```python
from build123d import *

# Parameters (mm, degrees)
F0_W      = 184.15
F0_H      = 50.8
F1_DEPTH  = 3.175
F3_D      = 3.2
F4_W      = 184.15
F4_H      = 3.175
F5_DEPTH  = 76.2
F7_D      = 3.3
F8_W      = 3.175
F8_H      = 47.625
F9_DEPTH  = 76.2
F10_W     = 19.05
F10_H     = 34.925
F11_DEPTH = 3.175
F12_W     = 3.175
F12_H     = 47.625
F13_DEPTH = 76.2
F14_W     = 13.2291666667
F14_H     = 31.75
F14_W_2   = 11.6416666667
F15_DEPTH = 3.175
F16_W     = 6.35
F16_H     = 6.35
F17_DEPTH = 6.35
F19_D     = 2.4
F19_DEPTH = 12.7
F19_TIP   = 0.7210327428
F20_W     = 121.4
F20_H     = 34.925
F21_DEPTH = 25.4
F22_W     = 60.2
F22_H     = 32.26
F23_DEPTH = 25.4
F24_W     = 177.8
F24_H     = 76.2
F25_DEPTH = 50.801
F26_W     = 6.35
F26_H     = 6.35
F27_DEPTH = 9.525
F28_D     = 2.4
F28_DEPTH = 12.7
F28_TIP   = 0.7210327428
F29_W     = 165.1
F29_H     = 6.35
F29_R     = 1.2
F30_DEPTH = 3.175


with BuildPart() as f1:
    # F0 (on Top) → F1 (new body)
    with BuildSketch(Plane.XY):
        with Locations((-3.8965528874, 0)):
            Rectangle(F0_W, F0_H)
    extrude(amount=F1_DEPTH)

    # F3 (through all)
    with Locations(Plane.XY.offset(3.175)):
        with Locations((-78.8965528874, 9.525), (-78.8965528874, -15.475), (71.1034471126, -15.475), (71.1034471126, 9.525)):
            Hole(F3_D / 2)

    # F4 (on face) → F5 (join)
    with BuildSketch(Plane.XY.offset(3.175)):
        with Locations((-3.8965528874, 23.8125)):
            Rectangle(F4_W, F4_H)
    extrude(amount=F5_DEPTH)

    # F7 (through all)
    with Locations(Plane.XZ.offset(-22.225)):
        with Locations((-70.5715528874, 66.675), (11.9784471126, 66.675), (10.7084471126, 18.415), (-64.2215528874, 18.415)):
            Hole(F7_D / 2)

    # F8 (on face) → F9 (join)
    with BuildSketch(Plane.XY.offset(3.175)):
        with Locations((-94.3840528874, -1.5875)):
            Rectangle(F8_W, F8_H)
    extrude(amount=F9_DEPTH)

    # F10 (on face) → F11 (cut, through all)
    with BuildSketch(Plane(origin=(-95.9715528874, 0, 0), x_dir=(0, -1, 0), z_dir=(-1, 0, 0))):
        with Locations((12.7, 58.7375)):
            Rectangle(F10_W, F10_H)
        with Locations((12.7, 20.6375)):
            Rectangle(F10_W, F10_H)
    extrude(amount=-F11_DEPTH, mode=Mode.SUBTRACT)

    # F12 (on face) → F13 (join)
    with BuildSketch(Plane.XY.offset(3.175)):
        with Locations((86.5909471126, -1.5875)):
            Rectangle(F12_W, F12_H)
    extrude(amount=F13_DEPTH)

    # F14 (on face) → F15 (cut, through all)
    with BuildSketch(Plane.YZ.offset(88.1784471126)):
        with Locations((-15.6104166667, 19.05)):
            Rectangle(F14_W, F14_H)
        with Locations((0, 19.05)):
            Rectangle(F14_W_2, F14_H)
        with Locations((15.6104166667, 19.05)):
            Rectangle(F14_W, F14_H)
    extrude(amount=-F15_DEPTH, mode=Mode.SUBTRACT)

    # F16 (on face) → F17 (join)
    with BuildSketch(Plane.XZ.offset(-22.225)):
        with Locations((-89.6215528874, 76.2)):
            Rectangle(F16_W, F16_H)
        with Locations((81.8284471126, 76.2)):
            Rectangle(F16_W, F16_H)
    extrude(amount=F17_DEPTH)

    # F19
    with Locations(Plane.XY.offset(79.375)):
        with Locations((-89.6215528874, 19.05), (81.8284471126, 19.05)):
            Hole(F19_D / 2, depth=F19_DEPTH)
            with Locations((0, 0, -(F19_DEPTH + F19_TIP / 2))):  # 118° drill point
                Cone(0, F19_D / 2, F19_TIP, mode=Mode.SUBTRACT)

    # F20 (on face) → F21 (cut)
    with BuildSketch(Plane.XY.offset(3.175)):
        with Locations((-3.8965528874, -1.5875)):
            Rectangle(F20_W, F20_H)
    extrude(amount=-F21_DEPTH, mode=Mode.SUBTRACT)

    # F22 (on face) → F23 (cut)
    with BuildSketch(Plane.XZ.offset(-22.225)):
        with Locations((-26.1215528874, 42.545)):
            Rectangle(F22_W, F22_H)
    extrude(amount=-F23_DEPTH, mode=Mode.SUBTRACT)

    # F24 (on face) → F25 (cut, through all)
    with BuildSketch(Plane.XZ.offset(25.4)):
        with Locations((-3.8965528874, 41.275)):
            Rectangle(F24_W, F24_H)
        Polygon((88.1784471126, 79.375), (85.0034471126, 79.375), (85.0034471126, 3.175), (85.0034471126, 0), (88.1784471126, 0), align=None)
    extrude(amount=-F25_DEPTH, mode=Mode.SUBTRACT)

    # F26 (on face) → F27 (join)
    with BuildSketch(Plane(origin=(0, 25.4, 0), x_dir=(-1, 0, 0), z_dir=(0, 1, 0))):
        with Locations((-81.8284471126, 6.35)):
            Rectangle(F26_W, F26_H)
        Polygon((-78.6534471126, 3.175), (-85.0034471126, 3.175), (-85.0034471126, 0), (95.9715528874, 0), (95.9715528874, 79.375), (92.7965528874, 79.375), (92.7965528874, 9.525), (92.7965528874, 3.175), (86.4465528874, 3.175), align=None)
        with Locations((89.6215528874, 6.35)):
            Rectangle(F26_W, F26_H)
    extrude(amount=-F27_DEPTH)

    # F28
    with Locations(Plane(origin=(0, 25.4, 0), x_dir=(-1, 0, 0), z_dir=(0, 1, 0))):
        with Locations((89.6215528874, 6.35), (-81.8284471126, 6.35)):
            Hole(F28_D / 2, depth=F28_DEPTH)
            with Locations((0, 0, -(F28_DEPTH + F28_TIP / 2))):  # 118° drill point
                Cone(0, F28_D / 2, F28_TIP, mode=Mode.SUBTRACT)

    # F29 (on face) → F30 (cut)
    with BuildSketch(Plane(origin=(0, 25.4, 0), x_dir=(-1, 0, 0), z_dir=(0, 1, 0))):
        with Locations((3.8965528874, 6.35)):
            Rectangle(F29_W, F29_H)
        Polygon((-78.6534471126, 9.525), (-85.0034471126, 9.525), (-85.0034471126, 2.9308686499), (92.7965528874, 2.9308686499), (92.7965528874, 9.525), (86.4465528874, 9.525), (86.4465528874, 3.175), (-78.6534471126, 3.175), align=None)
        with Locations((-81.8284471126, 6.35)):
            Circle(F29_R, mode=Mode.SUBTRACT)
        with Locations((89.6215528874, 6.35)):
            Circle(F29_R, mode=Mode.SUBTRACT)
    extrude(amount=-F30_DEPTH, mode=Mode.SUBTRACT)


solid = f1.part
```
Design review of the part built by this model. Coordinates are the model's own, in mm. A direction names the side the tool comes from. Round coordinates to 2 decimals unless told otherwise and drop trailing zeros. Write each loop counter-clockwise with the first axis right and the second up, starting at its lowest first coordinate (ties: lowest second). Pieces come first, ordered by that corner, then holes. Notation, with made-up numbers: (74, 89) -> (133, 89) arc R20 ccw to (133, 94) -> close; hole circle Ø3 at (30.5, 32). An arc over 180 degrees is marked (long way). Write item = value, one per line. Start each with the question number.
1) Clearance check with flat-ended pins moving along their axes: pin 1 (7 mm diameter, centred on x = 83, z = 7.5, fed in from -Y) (3 decimals); pin 2 (7 mm diameter, centred on x = 81, y = 18, fed in from +Z) (3 decimals); pin 3 (5 mm diameter, centred on x = -6, y = -20, fed in from +Z) (3 decimals). State where each tip first meets the part, or that it passes through.
2) Take a section at A-A, the plane y = 1. State the section outline as (x, z) points (3 decimals), plus the area to 3 significant figures.
3) Take a section at B-B, the plane z = 66. State the section outline as (x, y) points (3 decimals), plus the area to 3 significant figures.
4) Take a section at C-C, the plane y = -7.5. State the section outline as (x, z) points (3 decimals), plus the area to 3 significant figures.
5) Take a section at D-D, the plane x = -7. State the section outline as (y, z) points (3 decimals).
6) Mouldability with a two-part tool opening along Y and no side actions: class faces 1 (the face through (-94, -13, 76.2)), 2 (the face through (-5, 25.4, 2)), 3 (the face through (-46, -25.4, 1)), 4 (the face through (-90, 19, 9.525)) as +Y half, -Y half, draft (parallel to the pull), parting line (faces both ways), or undercut.
7) Tool access review of faces 5 (the face through (-90, 15.875, 5)), 6 (the face through (78.653, 19, 6)), 7 (the face through (85.003, 6, 3)), 8 (the face through (-5, 15.875, 2)), 9 (the face through (-94, -13, 41.275)): name each direction out of +Z, -Z, +X, -X, +Y, -Y from which nothing blocks a thin tool from reaching the whole face with its end or side.
8) Wall thickness on probe 1 along X at (y, z) = (17, 33.5); probe 2 along X at (y, z) = (17, 6); probe 3 along Z at (x, y) = (-68, 13) (3 decimals): over which ranges is each line inside the solid? List them lowest first. Write a range as from..to.
Results list:
q1.pin_1 = 15.875
q1.pin_2 = 9.525
q1.pin_3 = 3.175
q2.outline = (-95.972, 0) -> (-64.597, 0) -> (-64.597, 3.175) -> (-92.797, 3.175) -> (-92.797, 79.375) -> (-95.972, 79.375) -> close; (56.803, 0) -> (85.003, 0) -> (85.003, 3.175) -> (56.803, 3.175) -> close
q2.area = 431 mm²
q3.outline = (-95.972, -25.4) -> (-92.797, -25.4) -> (-92.797, -22.225) -> (-95.972, -22.225) -> close; (-95.972, -3.175) -> (-92.797, -3.175) -> (-92.797, 25.4) -> (-95.972, 25.4) -> close
q3.area = 101 mm²
q4.outline = (-95.972, 0) -> (-64.597, 0) -> (-64.597, 3.175) -> (-95.972, 3.175) -> close; (-95.972, 38.1) -> (-92.797, 38.1) -> (-92.797, 41.275) -> (-95.972, 41.275) -> close; (-95.972, 76.2) -> (-92.797, 76.2) -> (-92.797, 79.375) -> (-95.972, 79.375) -> close; (56.803, 0) -> (85.003, 0) -> (85.003, 3.175) -> (56.803, 3.175) -> close
q4.area = 209 mm²
q5.outline = (-25.4, 0) -> (-19.05, 0) -> (-19.05, 3.175) -> (-25.4, 3.175) -> close; (15.875, 0) -> (25.4, 0) -> (25.4, 2.931) -> (22.225, 2.931) -> (22.225, 3.175) -> (15.875, 3.175) -> close
q6.face_1 = undercut
q6.face_2 = +Y half
q6.face_3 = -Y half
q6.face_4 = draft
q7.face_5 = +Z, +X, -Y
q7.face_6 = +Z, +Y, -Y
q7.face_7 = +Z, -Z, +X, +Y, -Y
q7.face_8 = +Z, -Z
q7.face_9 = +X, -X
q8.probe_1 = -95.97..-92.8
q8.probe_2 = -95.97..-90.77, -88.47..-86.45, 78.65..80.68, 82.98..85
q8.probe_3 = 0..3.175
